Source: CAD feature listing. Evaluate the final solid. Frame: model axes, mm. Face numbers are marked on the shaded views. Round coordinates to 2 decimals unless told otherwise and drop trailing zeros. Write each loop counter-clockwise with the first axis right and the second up, starting at its lowest first coordinate (ties: lowest second). Pieces come first, ordered by that corner, then holes.
from build123d import *

# Parameters (mm, degrees)
SKETCH_1_R      = 20
EXTRUDE_1_DEPTH = 60
SKETCH_2_R      = 10
EXTRUDE_2_DEPTH = 5


with BuildPart() as part:
    # 草图1 → 凸台-拉伸1 (new body)
    with BuildSketch(Plane.XY):
        Circle(SKETCH_1_R)
    extrude(amount=EXTRUDE_1_DEPTH)

    # 草图2 → 凸台-拉伸2 (add)
    with BuildSketch(Plane.XY.offset(60)):
        Circle(SKETCH_2_R)
    extrude(amount=EXTRUDE_2_DEPTH)

    # 草图3 → 旋转1 (revolve)
    with BuildSketch(Plane(origin=(0, 0, 0), x_dir=(0, 0, -1), z_dir=(1, 0, 0)), mode=Mode.PRIVATE) as revolve_1_sk:
        with BuildLine():
            Line((-65, 0), (-75, 0))
            Line((-75, 0), (-75, 30))
            ThreePointArc((-75, 30), (-70, 35), (-65, 30))
            Line((-65, 30), (-65, 0))
        make_face()
    revolve(revolve_1_sk.sketch.rotate(Axis((0, 0, 65), (0, 0, 1)), 90), axis=Axis((0, 0, 65), (0, 0, 1)))


solid = part.part
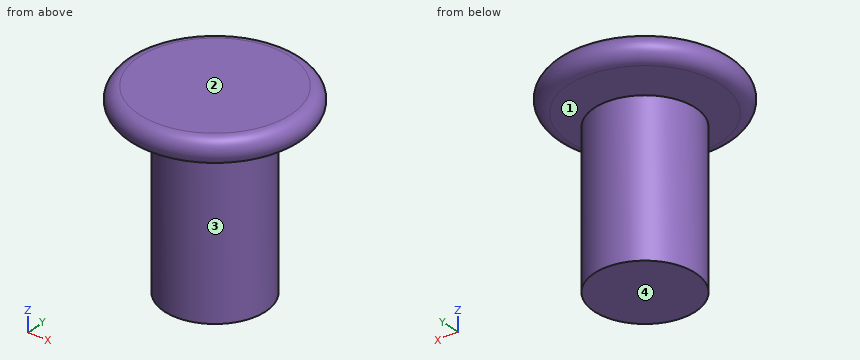
1) Section query C-C on z = 62. Return the cut outline in (x, y), then the cut area to 3 significant figures.
Taken from the geometry:
outline: circle Ø20 at (0, 0)
area: 314 mm2
2) Pull-direction query (Z, two-part tool) for the marked faces 1, 2, 3 and 4; classes: released by +Z, released by -Z, zero draft, split by the parting line, or undercut.
Taken from the geometry:
face 1: undercut
face 2: released by +Z
face 3: zero draft
face 4: released by -Z
3) Section query A-A on x = 0. Return the cut outline in (y, z).
Taken from the geometry:
outline: (-30, 65) - (-10, 65) - (-10, 60) - (-20, 60) - (-20, 0) - (20, 0) - (20, 60) - (10, 60) - (10, 65) - (30, 65) arc R5 ccw to (30, 75) - (-30, 75) arc R5 ccw to start
4) Material intervals for line 1 (Z direction, x = -14.5, y = 7.5); line 2 (Z direction, x = -14, y = -22.5); line 3 (Y direction, x = 16.5, z = 59), sorted ascending.
Taken from the geometry:
line 1: z = 0 to 60, 65 to 75
line 2: z = 65 to 75
line 3: y = -11.3 to 11.3
5) Section query D-D on z = 14. Return the cut outline in (x, y).
Taken from the geometry:
outline: circle Ø40 at (0, 0)
6) Contact query for flat-ended pins moving along their axis: P1, Ø4, axis at y = -3.5, z = 49.5, coming from the -X side; P2, Ø3, axis at y = 15, z = 24, coming from the +X side; P3, Ø8, axis at x = 19.5, z = 35, coming from the -Y side. Output: stop coordinate, or through.
Taken from the geometry:
P1: stops at x = -19.94
P2: stops at x = 14.76
P3: stops at y = -12.64
